from build123d import *

# Parameters (mm, degrees)
BOSS_EXTRU_1_DEPTH      = 6
ESQUISSE4_R             = 20
ESQUISSE4_R_2           = 14.95
ENL_V_MAT_EXTRU_2_DEPTH = 3
ESQUISSE5_W             = 16.42
ESQUISSE5_H             = 20
BOSS_EXTRU_2_DEPTH      = 6
ESQUISSE6_R             = 1.5
ENL_V_MAT_EXTRU_3_DEPTH = 10
ESQUISSE9_R             = 1.5
ENL_V_MAT_EXTRU_4_DEPTH = 10


with BuildPart() as part:
    # Esquisse1 → Boss.-Extru.1 (new body)
    with BuildSketch(Plane.XY):
        with BuildLine():
            ThreePointArc((52.992232765, 28.099272116), (32.992232765, 48.099272116), (12.992232765, 28.099272116))
            Line((12.992232765, 28.099272116), (32.992232765, 28.099272116))
            Line((32.992232765, 28.099272116), (32.992232765, 8.099272116))
            ThreePointArc((32.992232765, 8.099272116), (47.134368389, 13.957136493), (52.992232765, 28.099272116))
        make_face()
        with BuildLine():
            Line((32.992232765, 28.099272116), (12.992232765, 28.099272116))
            ThreePointArc((12.992232765, 28.099272116), (18.850097141, 13.957136493), (32.992232765, 8.099272116))
            Line((32.992232765, 8.099272116), (32.992232765, 28.099272116))
        make_face()
        with BuildLine():
            Line((12.992232765, 28.099272116), (-45.58279523, 28.099272116))
            Line((-45.58279523, 28.099272116), (-45.58279523, 8.099272116))
            Line((-45.58279523, 8.099272116), (32.992232765, 8.099272116))
            ThreePointArc((32.992232765, 8.099272116), (18.850097141, 13.957136493), (12.992232765, 28.099272116))
        make_face()
    extrude(amount=BOSS_EXTRU_1_DEPTH)

    # Esquisse4 → Enlèv. mat.-Extru.2 (cut)
    with BuildSketch(Plane.XY.offset(6)):
        with Locations((32.992232765, 28.099272116)):
            Circle(ESQUISSE4_R)
        with Locations((32.992232765, 28.099272116)):
            Circle(ESQUISSE4_R_2, mode=Mode.SUBTRACT)
    extrude(amount=-ENL_V_MAT_EXTRU_2_DEPTH, mode=Mode.SUBTRACT)

    # Esquisse5 → Boss.-Extru.2 (add)
    with BuildSketch(Plane.XY.offset(6)):
        with Locations((-53.79279523, 18.099272116)):
            Rectangle(ESQUISSE5_W, ESQUISSE5_H)
    extrude(amount=-BOSS_EXTRU_2_DEPTH)

    # Esquisse6 → Enlèv. mat.-Extru.3 (cut)
    with BuildSketch(Plane.XY.offset(6)):
        with Locations((32.992232765, 41.099272116)):
            Circle(ESQUISSE6_R)
        with Locations((45.992232765, 28.099272116)):
            Circle(ESQUISSE6_R)
        with Locations((32.992232765, 15.099272116)):
            Circle(ESQUISSE6_R)
        with Locations((19.992232765, 28.099272116)):
            Circle(ESQUISSE6_R)
    extrude(amount=-ENL_V_MAT_EXTRU_3_DEPTH, mode=Mode.SUBTRACT)

    # Esquisse9 → Enlèv. mat.-Extru.4 (cut)
    with BuildSketch(Plane(origin=(0, 0, 0), x_dir=(-1, 0, 0), z_dir=(0, 0, -1))):
        with Locations((59.00279523, 25.099272116)):
            Circle(ESQUISSE9_R)
        with Locations((59.00279523, 11.099272116)):
            Circle(ESQUISSE9_R)
    extrude(amount=-ENL_V_MAT_EXTRU_4_DEPTH, mode=Mode.SUBTRACT)


solid = part.part
The listing builds one solid part. Answer for the finished solid, in the listing's coordinates (mm). A direction names the side the tool comes from. Give positions to 0.01 mm unless a question says otherwise; leave off trailing zeros. Order: outer loops, then holes, each group sorted by start corner. A loop starts at its lowest first (then second) coordinate and runs counter-clockwise, first axis right, second up. Notation, with made-up numbers: (-32.5, -4) -> (-19.5, -4) arc R13 ccw to (-19.5, 21) -> close; hole circle Ø9 at (32.25, 89.25). An arc over 180 degrees is marked (long way). Put each result on its own line as item: value.
Item 1: Given P1, Ø3.5, axis at x = 45.99, y = 28.1, coming from the +Z side; P2, Ø1.8, axis at x = -9.5, z = 2, coming from the +Y side; P3, Ø1.5, axis at y = 17.5, z = 0.5, coming from the +X side; P4, Ø2, axis at y = 32.5, z = 1.5, coming from the -X side, each flat-ended and moving along its own axis, determine where each tip first touches the part or whether it passes through.
Established:
P1: stops at z = 6
P2: stops at y = 28.1
P3: stops at x = 50.4
P4: stops at x = 13.28
Item 2: For faces 1 (the face through (-25, 28.099, 3)), 2 (the face through (33, 28, 6)), 3 (the face through (31.046, 42.922, 4.521)), determine the directions among +Z, -Z, +X, -X, +Y, -Y from which every point of the face is accessible in a straight line to the end or side of a thin tool.
Established:
face 1: +Z, -Z, -X, +Y
face 2: +Z, +X, -X, +Y, -Y
face 3: +Z
Item 3: A cutting plane is placed at C-C on x = -20. Give the vertices of the cut face in (y, z).
Established:
outline: (8.1, 0) -> (28.1, 0) -> (28.1, 6) -> (8.1, 6) -> close
Item 4: Straight lines are drawn through the part: line 1 (Y direction, x = -29, z = 4.05); line 2 (Z direction, x = 47, y = 17); line 3 (Y direction, x = 26.5, z = 5.55). For each, find the intervals that lie inside material, in ascending order.
Established:
line 1: y = 8.1 to 28.1
line 2: z = 0 to 3
line 3: y = 8.1 to 9.18, 14.63 to 41.57
Item 5: A cutting plane is placed at A-A on z = 4.75. Give the vertices of the cut face in (x, y), plus the area to 3 significant figures.
Established:
outline: (-62, 8.1) -> (32.99, 8.1) arc R20 cw to (12.99, 28.1) -> (-62, 28.1) -> close; circle Ø29.9 at (32.99, 28.1); hole circle Ø3 at (-59, 11.1); hole circle Ø3 at (-59, 25.1); hole circle Ø3 at (19.99, 28.1); hole circle Ø3 at (32.99, 15.1); hole circle Ø3 at (32.99, 41.1); hole circle Ø3 at (45.99, 28.1)
area: 2,250 mm^2
Item 6: A cutting plane is placed at B-B on x = 20.5. Give the vertices of the cut face in (y, z).
Established:
outline: (8.1, 0) -> (26.69, 0) -> (26.69, 6) -> (19.89, 6) -> (19.89, 3) -> (12.48, 3) -> (12.48, 6) -> (8.1, 6) -> close; (29.51, 0) -> (43.72, 0) -> (43.72, 3) -> (36.31, 3) -> (36.31, 6) -> (29.51, 6) -> close
Item 7: A cutting plane is placed at D-D on y = 37.5. Give the vertices of the cut face in (x, z).
Established:
outline: (15.34, 0) -> (50.65, 0) -> (50.65, 3) -> (44.62, 3) -> (44.62, 6) -> (21.37, 6) -> (21.37, 3) -> (15.34, 3) -> close
Item 8: For a pull along X with two mould halves and no side action, classify faces 4 (the face through (34.378, 40.525, 3.042)), 5 (the face through (-62.003, 18, 3)), 6 (the face through (-15, 8.099, 3)) as released by +X, released by -X, zero draft, split by the parting line, or undercut.
Established:
face 4: undercut
face 5: released by -X
face 6: zero draft
